Here's how the part is built. I have some questions about the finished solid (model axes, mm). Give positions to 0.01 mm unless a question says otherwise; leave off trailing zeros. Write each loop counter-clockwise with the first axis right and the second up, starting at its lowest first coordinate (ties: lowest second). Pieces come first, ordered by that corner, then holes. Notation, with made-up numbers: (1.25, 83.25) -> (18.25, 83.25) arc R19 cw to (18.25, 106.25) -> close; hole circle Ø2 at (-4.5, 42). An arc over 180 degrees is marked (long way). Return JSON: item names as keys, results as strings.
from build123d import *

# Parameters (mm, degrees)
SKETCH_1_W          = 270
SKETCH_1_H          = 5
EXTRUDE_1_DEPTH     = 95
SKETCH_2_R          = 2.25
SKETCH_2_R_2        = 17.5
CUT_EXTRUDE_1_DEPTH = 10
SKETCH_3_W          = 70
SKETCH_3_H          = 20
CUT_EXTRUDE_2_DEPTH = 10
SKETCH_6_W          = 219.864116777
SKETCH_6_H          = 129.686347052
CUT_EXTRUDE_5_DEPTH = 10
SKETCH_7_W          = 55.982845341
SKETCH_7_H          = 55
EXTRUDE_1_2_DEPTH   = 5
SKETCH_9_R          = 2
CUT_EXTRUDE_6_DEPTH = 5
FILLET_1_R          = 5
CUT_EXTRUDE_START   = -5
CUT_EXTRUDE_7_DEPTH = 5
FILLET_2_R          = 5


with BuildPart() as part:
    # 草图1 → Extrude 1 (new body)
    with BuildSketch(Plane.XY):
        with Locations((-135, -2.5)):
            Rectangle(SKETCH_1_W, SKETCH_1_H)
    extrude(amount=EXTRUDE_1_DEPTH)

    # 草图2 → 切除-拉伸1 (cut)
    with BuildSketch(Plane(origin=(0, 0, 0), x_dir=(1, 0, 0), z_dir=(0, 1, 0))):
        with Locations(Location((-246, -25.75, 0), (0, 0, 270))):
            Circle(SKETCH_2_R)
        with Locations(Location((-229.338533362, -33.519369489, 0), (0, 0, 270))):
            Circle(SKETCH_2_R)
        with Locations(Location((-262.661466638, -33.519369489, 0), (0, 0, 270))):
            Circle(SKETCH_2_R)
        with Locations(Location((-262.661466638, -61.480630511, 0), (0, 0, 270))):
            Circle(SKETCH_2_R)
        with Locations(Location((-246, -69.25, 0), (0, 0, 270))):
            Circle(SKETCH_2_R)
        with Locations(Location((-229.338533362, -61.480630511, 0), (0, 0, 270))):
            Circle(SKETCH_2_R)
        with Locations(Location((-246, -47.5, 0), (0, 0, 270))):
            Circle(SKETCH_2_R_2)
    extrude(amount=-CUT_EXTRUDE_1_DEPTH, mode=Mode.SUBTRACT)

    # 草图3 → 切除-拉伸2 (cut)
    with BuildSketch(Plane(origin=(0, 0, 0), x_dir=(1, 0, 0), z_dir=(0, 1, 0))):
        with Locations((-235, -85)):
            Rectangle(SKETCH_3_W, SKETCH_3_H)
        with Locations((-235, -10)):
            Rectangle(SKETCH_3_W, SKETCH_3_H)
        with BuildLine():
            Line((-190, -10), (-190, -34.757359313))
            ThreePointArc((-190, -34.757359313), (-188.148050297, -37.52899791), (-184.878679656, -36.878679656))
            Line((-184.878679656, -36.878679656), (-160.121320344, -12.121320344))
            ThreePointArc((-160.121320344, -12.121320344), (-159.47100209, -8.851949703), (-162.242640687, -7))
            Line((-162.242640687, -7), (-187, -7))
            ThreePointArc((-187, -7), (-189.121320344, -7.878679656), (-190, -10))
        make_face()
        with BuildLine():
            Line((-154.121320344, -12.121320344), (-178.878679656, -36.878679656))
            ThreePointArc((-178.878679656, -36.878679656), (-179.52899791, -40.148050297), (-176.757359313, -42))
            Line((-176.757359313, -42), (-152, -42))
            ThreePointArc((-152, -42), (-149.878679656, -41.121320344), (-149, -39))
            Line((-149, -39), (-149, -14.242640687))
            ThreePointArc((-149, -14.242640687), (-150.851949703, -11.47100209), (-154.121320344, -12.121320344))
        make_face()
        with BuildLine():
            Line((-112.242640687, -7), (-137, -7))
            ThreePointArc((-137, -7), (-139.121320344, -7.878679656), (-140, -10))
            Line((-140, -10), (-140, -34.757359313))
            ThreePointArc((-140, -34.757359313), (-138.148050297, -37.52899791), (-134.878679656, -36.878679656))
            Line((-134.878679656, -36.878679656), (-110.121320344, -12.121320344))
            ThreePointArc((-110.121320344, -12.121320344), (-109.47100209, -8.851949703), (-112.242640687, -7))
        make_face()
        with BuildLine():
            Line((-99, -39), (-99, -14.242640687))
            ThreePointArc((-99, -14.242640687), (-100.851949703, -11.47100209), (-104.121320344, -12.121320344))
            Line((-104.121320344, -12.121320344), (-128.878679656, -36.878679656))
            ThreePointArc((-128.878679656, -36.878679656), (-129.52899791, -40.148050297), (-126.757359313, -42))
            Line((-126.757359313, -42), (-102, -42))
            ThreePointArc((-102, -42), (-99.878679656, -41.121320344), (-99, -39))
        make_face()
        with BuildLine():
            Line((-112.242640687, -52), (-137, -52))
            ThreePointArc((-137, -52), (-139.121320344, -52.878679656), (-140, -55))
            Line((-140, -55), (-140, -79.757359313))
            ThreePointArc((-140, -79.757359313), (-138.148050297, -82.52899791), (-134.878679656, -81.878679656))
            Line((-134.878679656, -81.878679656), (-110.121320344, -57.121320344))
            ThreePointArc((-110.121320344, -57.121320344), (-109.47100209, -53.851949703), (-112.242640687, -52))
        make_face()
        with BuildLine():
            Line((-99, -84), (-99, -59.242640687))
            ThreePointArc((-99, -59.242640687), (-100.851949703, -56.47100209), (-104.121320344, -57.121320344))
            Line((-104.121320344, -57.121320344), (-128.878679656, -81.878679656))
            ThreePointArc((-128.878679656, -81.878679656), (-129.52899791, -85.148050297), (-126.757359313, -87))
            Line((-126.757359313, -87), (-102, -87))
            ThreePointArc((-102, -87), (-99.878679656, -86.121320344), (-99, -84))
        make_face()
        with BuildLine():
            Line((-162.242640687, -52), (-187, -52))
            ThreePointArc((-187, -52), (-189.121320344, -52.878679656), (-190, -55))
            Line((-190, -55), (-190, -79.757359313))
            ThreePointArc((-190, -79.757359313), (-188.148050297, -82.52899791), (-184.878679656, -81.878679656))
            Line((-184.878679656, -81.878679656), (-160.121320344, -57.121320344))
            ThreePointArc((-160.121320344, -57.121320344), (-159.47100209, -53.851949703), (-162.242640687, -52))
        make_face()
        with BuildLine():
            Line((-149, -84), (-149, -59.242640687))
            ThreePointArc((-149, -59.242640687), (-150.851949703, -56.47100209), (-154.121320344, -57.121320344))
            Line((-154.121320344, -57.121320344), (-178.878679656, -81.878679656))
            ThreePointArc((-178.878679656, -81.878679656), (-179.52899791, -85.148050297), (-176.757359313, -87))
            Line((-176.757359313, -87), (-152, -87))
            ThreePointArc((-152, -87), (-149.878679656, -86.121320344), (-149, -84))
        make_face()
        with BuildLine():
            Line((-62.242640687, -7), (-87, -7))
            ThreePointArc((-87, -7), (-89.121320344, -7.878679656), (-90, -10))
            Line((-90, -10), (-90, -34.757359313))
            ThreePointArc((-90, -34.757359313), (-88.148050297, -37.52899791), (-84.878679656, -36.878679656))
            Line((-84.878679656, -36.878679656), (-60.121320344, -12.121320344))
            ThreePointArc((-60.121320344, -12.121320344), (-59.47100209, -8.851949703), (-62.242640687, -7))
        make_face()
        with BuildLine():
            Line((-49, -39), (-49, -14.242640687))
            ThreePointArc((-49, -14.242640687), (-50.851949703, -11.47100209), (-54.121320344, -12.121320344))
            Line((-54.121320344, -12.121320344), (-78.878679656, -36.878679656))
            ThreePointArc((-78.878679656, -36.878679656), (-79.52899791, -40.148050297), (-76.757359313, -42))
            Line((-76.757359313, -42), (-52, -42))
            ThreePointArc((-52, -42), (-49.878679656, -41.121320344), (-49, -39))
        make_face()
        with BuildLine():
            Line((-62.242640687, -52), (-87, -52))
            ThreePointArc((-87, -52), (-89.121320344, -52.878679656), (-90, -55))
            Line((-90, -55), (-90, -79.757359313))
            ThreePointArc((-90, -79.757359313), (-88.148050297, -82.52899791), (-84.878679656, -81.878679656))
            Line((-84.878679656, -81.878679656), (-60.121320344, -57.121320344))
            ThreePointArc((-60.121320344, -57.121320344), (-59.47100209, -53.851949703), (-62.242640687, -52))
        make_face()
        with BuildLine():
            Line((-49, -84), (-49, -59.242640687))
            ThreePointArc((-49, -59.242640687), (-50.851949703, -56.47100209), (-54.121320344, -57.121320344))
            Line((-54.121320344, -57.121320344), (-78.878679656, -81.878679656))
            ThreePointArc((-78.878679656, -81.878679656), (-79.52899791, -85.148050297), (-76.757359313, -87))
            Line((-76.757359313, -87), (-52, -87))
            ThreePointArc((-52, -87), (-49.878679656, -86.121320344), (-49, -84))
        make_face()
    extrude(amount=-CUT_EXTRUDE_2_DEPTH, mode=Mode.SUBTRACT)

    # 草图6 → 切除-拉伸5 (cut)
    with BuildSketch(Plane(origin=(0, 0, 0), x_dir=(1, 0, 0), z_dir=(0, 1, 0))):
        with Locations((-104.085096271, -53.191913683)):
            Rectangle(SKETCH_6_W, SKETCH_6_H)
    extrude(amount=-CUT_EXTRUDE_5_DEPTH, mode=Mode.SUBTRACT)

    # 草图7 → Extrude 1 2 (add)
    with BuildSketch(Plane(origin=(0, 0, 0), x_dir=(1, 0, 0), z_dir=(0, 1, 0))):
        with BuildLine():
            Line((-246, -7.5), (-166, -7.5))
            Line((-166, -7.5), (-166, -87.5))
            Line((-166, -87.5), (-246, -87.5))
            ThreePointArc((-246, -87.5), (-286, -47.5), (-246, -7.5))
        make_face()
        with Locations((-242.008577329, -47.5)):
            Rectangle(SKETCH_7_W, SKETCH_7_H, mode=Mode.SUBTRACT)
    extrude(amount=-EXTRUDE_1_2_DEPTH)

    # 草图9 → 切除-拉伸6 (cut)
    with BuildSketch(Plane(origin=(0, 0, 0), x_dir=(1, 0, 0), z_dir=(0, 1, 0))):
        with Locations(Location((-192, -27.5, 0), (0, 0, 270))):
            Circle(SKETCH_9_R)
        with Locations(Location((-174, -27.5, 0), (0, 0, 270))):
            Circle(SKETCH_9_R)
        with Locations(Location((-174, -40.833333333, 0), (0, 0, 270))):
            Circle(SKETCH_9_R)
        with Locations(Location((-174, -54.166666667, 0), (0, 0, 270))):
            Circle(SKETCH_9_R)
        with Locations(Location((-174, -67.5, 0), (0, 0, 270))):
            Circle(SKETCH_9_R)
        with Locations(Location((-192, -40.833333333, 0), (0, 0, 270))):
            Circle(SKETCH_9_R)
        with Locations(Location((-192, -54.166666667, 0), (0, 0, 270))):
            Circle(SKETCH_9_R)
        with Locations(Location((-192, -67.5, 0), (0, 0, 270))):
            Circle(SKETCH_9_R)
    extrude(amount=-CUT_EXTRUDE_6_DEPTH, mode=Mode.SUBTRACT)

    # 圆角1
    fillet_1_edges = [part.edges().sort_by_distance(p)[0] for p in [
        (-166, -2.5, 7.5),
        (-166, -2.5, 87.5),
    ]]
    fillet(fillet_1_edges, radius=FILLET_1_R)

    # 草图10 → 切除-拉伸7 (cut)
    with BuildSketch(Plane(origin=(0, 0, 0), x_dir=(1, 0, 0), z_dir=(0, 1, 0)).offset(CUT_EXTRUDE_START)):
        with BuildLine():
            Line((-171, -7.5), (-236.784609691, -7.5))
            Line((-236.784609691, -7.5), (-216, -19.5))
            Line((-216, -19.5), (-166, -19.5))
            Line((-166, -19.5), (-166, -12.5))
            ThreePointArc((-166, -12.5), (-167.464466094, -8.964466094), (-171, -7.5))
        make_face()
        with BuildLine():
            Line((-166, -82.5), (-166, -75.5))
            Line((-166, -75.5), (-216, -75.5))
            Line((-216, -75.5), (-236.784609691, -87.5))
            Line((-236.784609691, -87.5), (-171, -87.5))
            ThreePointArc((-171, -87.5), (-167.464466094, -86.035533906), (-166, -82.5))
        make_face()
    extrude(amount=CUT_EXTRUDE_7_DEPTH, mode=Mode.SUBTRACT)

    # 圆角2
    fillet_2_edges = [part.edges().sort_by_distance(p)[0] for p in [
        (-216, -2.5, 19.5),
        (-166, -2.5, 19.5),
        (-216, -2.5, 75.5),
        (-166, -2.5, 75.5),
    ]]
    fillet(fillet_2_edges, radius=FILLET_2_R)


solid = part.part
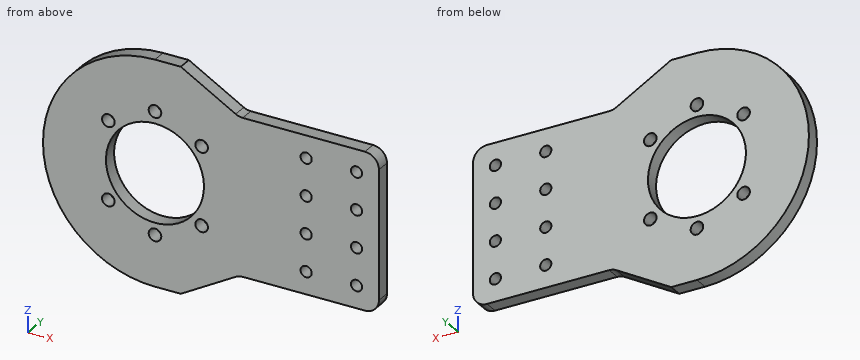
1. Suppose I cut it at B-B, the plane z = 47.5. List the corners of the cut face in (x, y) for me.
Taken from the geometry:
{"outline": "(-286, -5) -> (-263.5, -5) -> (-263.5, 0) -> (-286, 0) -> close; (-228.5, -5) -> (-166, -5) -> (-166, 0) -> (-228.5, 0) -> close"}
2. Suppose I cut it at D-D, the plane y = -4.15. Count the separate pieces of the cut face and the enclosed holes in it, and give its area (3 significant figures).
Taken from the geometry:
{"separate pieces": "1", "enclosed holes": "15", "area": "6,300 mm²"}
3. Suppose I cut it at C-C, the plane x = -250. List the corners of the cut face in (y, z) for me, and give its area (3 significant figures).
Taken from the geometry:
{"outline": "(-5, 7.7) -> (0, 7.7) -> (0, 30.46) -> (-5, 30.46) -> close; (-5, 64.54) -> (0, 64.54) -> (0, 87.3) -> (-5, 87.3) -> close", "area": "228 mm²"}
4. For pin 1 Ø3.5 at (x, z) = (-246, 25.75) entering from +Y; pin 2 Ø1 at (x, y) = (-188, -4) entering from -Z; pin 3 Ø1 at (x, y) = (-217.5, -2.5) entering from +Z, each with a flat end and sliding along its axis, tell me the tip position at first contact or that it passes through.
Taken from the geometry:
{"pin 1": "passes through", "pin 2": "stops at z = 19.5", "pin 3": "stops at z = 76.65"}
5. If I drill on line 1 (Z direction, x = -174, y = -1.95); line 2 (X direction, y = -0.45, z = 27); line 3 (X direction, y = -1.25, z = 47.5), over which ranges is the centre line in solid material (lowest first)? Write a range as [from, to].
Taken from the geometry:
{"line 1": "z = [19.5, 25.5], [29.5, 38.83], [42.83, 52.17], [56.17, 65.5], [69.5, 75.5]", "line 2": "x = [-280.35, -247.87], [-244.13, -193.94], [-190.06, -175.94], [-172.06, -166]", "line 3": "x = [-286, -263.5], [-228.5, -166]"}
6. Suppose I cut it at A-A, the plane x = -192. List the corners of the cut face in (y, z) for me, and give its area (3 significant figures).
Taken from the geometry:
{"outline": "(-5, 19.5) -> (0, 19.5) -> (0, 25.5) -> (-5, 25.5) -> close; (-5, 29.5) -> (0, 29.5) -> (0, 38.83) -> (-5, 38.83) -> close; (-5, 42.83) -> (0, 42.83) -> (0, 52.17) -> (-5, 52.17) -> close; (-5, 56.17) -> (0, 56.17) -> (0, 65.5) -> (-5, 65.5) -> close; (-5, 69.5) -> (0, 69.5) -> (0, 75.5) -> (-5, 75.5) -> close", "area": "200 mm²"}
